from build123d import *

# Parameters (mm, degrees)
SKETCH1_R           = 7
SKETCH1_W           = 10
SKETCH1_H           = 3
BOSS_EXTRUDE1_DEPTH = 3
FILLET1_R           = 0.5


with BuildPart() as part:
    # Sketch1 → Boss-Extrude1 (new body)
    with BuildSketch(Plane(origin=(0, 0, 0), x_dir=(1, 0, 0), z_dir=(0, 1, 0))):
        with BuildLine():
            Line((-23.198633067, -13), (6.801366933, -13))
            Line((6.801366933, -13), (6.801366933, 10))
            Line((6.801366933, 10), (9.801366933, 10))
            Line((9.801366933, 10), (9.801366933, 20))
            Line((9.801366933, 20), (6.801366933, 20))
            Line((6.801366933, 20), (6.801366933, 18.5))
            ThreePointArc((6.801366933, 18.5), (6.601366933, 17.5), (6.801366933, 16.5))
            Line((6.801366933, 16.5), (6.801366933, 15))
            Line((6.801366933, 15), (3.801366933, 15))
            Line((3.801366933, 15), (3.801366933, 16.5))
            ThreePointArc((3.801366933, 16.5), (4.001366933, 17.5), (3.801366933, 18.5))
            Line((3.801366933, 18.5), (3.801366933, 30))
            Line((3.801366933, 30), (9.801366933, 30))
            Line((9.801366933, 30), (9.801366933, 39))
            Line((9.801366933, 39), (6.801366933, 39))
            Line((6.801366933, 39), (6.801366933, 37.5))
            ThreePointArc((6.801366933, 37.5), (6.601366933, 36.5), (6.801366933, 35.5))
            Line((6.801366933, 35.5), (6.801366933, 34))
            Line((6.801366933, 34), (3.801366933, 34))
            Line((3.801366933, 34), (3.801366933, 35.5))
            ThreePointArc((3.801366933, 35.5), (4.001366933, 36.5), (3.801366933, 37.5))
            Line((3.801366933, 37.5), (3.801366933, 39))
            Line((3.801366933, 39), (-20.198633067, 39))
            Line((-20.198633067, 39), (-20.198633067, 37.5))
            ThreePointArc((-20.198633067, 37.5), (-20.398633067, 36.5), (-20.198633067, 35.5))
            Line((-20.198633067, 35.5), (-20.198633067, 34))
            Line((-20.198633067, 34), (-23.198633067, 34))
            Line((-23.198633067, 34), (-23.198633067, 35.5))
            ThreePointArc((-23.198633067, 35.5), (-22.998633067, 36.5), (-23.198633067, 37.5))
            Line((-23.198633067, 37.5), (-23.198633067, 39))
            Line((-23.198633067, 39), (-26.198633067, 39))
            Line((-26.198633067, 39), (-26.198633067, 30))
            Line((-26.198633067, 30), (-20.198633067, 30))
            Line((-20.198633067, 30), (-20.198633067, 18.5))
            ThreePointArc((-20.198633067, 18.5), (-20.398633067, 17.5), (-20.198633067, 16.5))
            Line((-20.198633067, 16.5), (-20.198633067, 15))
            Line((-20.198633067, 15), (-23.198633067, 15))
            Line((-23.198633067, 15), (-23.198633067, 16.5))
            ThreePointArc((-23.198633067, 16.5), (-22.998633067, 17.5), (-23.198633067, 18.5))
            Line((-23.198633067, 18.5), (-23.198633067, 20))
            Line((-23.198633067, 20), (-26.198633067, 20))
            Line((-26.198633067, 20), (-26.198633067, 10))
            Line((-26.198633067, 10), (-23.198633067, 10))
            Line((-23.198633067, 10), (-23.198633067, -13))
        make_face()
        with Locations(Location((-8.198633067, 22, 0), (0, 0, 270))):
            Circle(SKETCH1_R, mode=Mode.SUBTRACT)
        with Locations((-8.198633067, 34.5)):
            Rectangle(SKETCH1_W, SKETCH1_H, mode=Mode.SUBTRACT)
    extrude(amount=BOSS_EXTRUDE1_DEPTH)

    # Fillet1
    fillet1_edges = [part.edges().sort_by_distance(p)[0] for p in [
        (-23.198633067, 1.5, -39),
        (6.801366933, 1.5, -39),
        (6.801366933, 1.5, -20),
        (-23.198633067, 1.5, -20),
    ]]
    fillet(fillet1_edges, radius=FILLET1_R)


solid = part.part
The listing builds one solid part. Answer for the finished solid, in the listing's coordinates (mm). A direction names the side the tool comes from. Round coordinates to 2 decimals unless told otherwise and drop trailing zeros. Write each loop counter-clockwise with the first axis right and the second up, starting at its lowest first coordinate (ties: lowest second). Pieces come first, ordered by that corner, then holes. Notation, with made-up numbers: (24, 78) - (75, 78) arc R26 ccw to (75, 96) - close; hole circle Ø7 at (19, 52.5). An arc over 180 degrees is marked (long way). Use one line per item in the form item = value. Start each with the question number.
Item 1: A cutting plane is placed at D-D (y = 1.8). Give the number of separate pieces and of enclosed holes in the cut face, plus the area to 3 significant figures.
Item 2: A tool of negligible diameter and unlimited length cuts with its end or side. For faces 4 (the flat face through (-25, 1, -20)), 5 (the flat face through (6.801, 1, -38)), 6 (the flat face through (-23.199, 1, -16)), from which of +Z, -Z, +X, -X, +Y, -Y can it reach the whole face along a straight path? Write none if from no direction.
Item 3: A cutting plane is placed at C-C (x = -9.5). Write down the section's boundary in (y, z), plus the area to 3 significant figures.
Item 4: A cutting plane is placed at B-B (x = -21). Write down the section's boundary in (y, z), plus the area to 3 significant figures.
Item 5: A cutting plane is placed at A-A (z = -22). Write down the section's boundary in (x, y).
Item 6: Find the intervals of material crossed by line 1 (X direction, y = 2.4, z = -22); line 2 (Z direction, x = -5.5, y = 1.15); line 3 (Z direction, x = -21, y = 0.7), in increasing order. Write a range as [from, to].
Item 7: Flat-ended cylindrical pins translate along their axes: pin 1 Ø1.5 at (x, y) = (8.5, 2) entering from +Z; pin 2 Ø1.5 at (x, y) = (5, 1) entering from -Z. Find the tip coordinate at first contact, or state that the pin passes through.
Item 8: Determine the mould class of faces 1 (the flat face through (-20.199, 1, -35)), 2 (the flat face through (-25, 1, -39)), 3 (the flat face through (6.801, 1, 2)) for opening direction Z: +Z half, -Z half, draft (parallel to the pull), parting line (faces both ways), or undercut.
The answers:
q1.separate_pieces = 1
q1.enclosed_holes = 2
q1.area = 1,370 mm^2
q2.face_4 = -X, +Y, -Y
q2.face_5 = -Z, +Y, -Y
q2.face_6 = +Y, -Y
q3.outline = (0, -39) - (3, -39) - (3, -36) - (0, -36) - close; (0, -33) - (3, -33) - (3, -28.88) - (0, -28.88) - close; (0, -15.12) - (3, -15.12) - (3, 13) - (0, 13) - close
q3.area = 106 mm^2
q4.outline = (0, -34) - (3, -34) - (3, -30) - (0, -30) - close; (0, -15) - (3, -15) - (3, 13) - (0, 13) - close
q4.area = 96.0 mm^2
q5.outline = (-20.2, 0) - (-15.2, 0) - (-15.2, 3) - (-20.2, 3) - close; (-1.2, 0) - (3.8, 0) - (3.8, 3) - (-1.2, 3) - close
q6.line_1 = [-20.2, -15.2], [-1.2, 3.8]
q6.line_2 = [-39, -36], [-33, -28.46], [-15.54, 13]
q6.line_3 = [-34, -30], [-15, 13]
q7.pin_1 = -10
q7.pin_2 = -34
q8.face_1 = undercut
q8.face_2 = -Z half
q8.face_3 = draft
